from build123d import *

# Parameters (mm, degrees)
SKETCH1_W           = 16
SKETCH1_H           = 26
BOSS_EXTRUDE1_DEPTH = 3.5
SKETCH2_W           = 16
SKETCH2_H           = 26
BOSS_EXTRUDE2_DEPTH = 3.5
SKETCH3_R           = 5
CUT_EXTRUDE1_DEPTH  = 2.5


with BuildPart() as part:
    # Sketch1 → Boss-Extrude1 (new body)
    with BuildSketch(Plane.XY):
        with Locations((8, 13)):
            Rectangle(SKETCH1_W, SKETCH1_H)
        with BuildLine():
            Line((13.25, 23.790620927), (13.25, 2.209379073))
            ThreePointArc((13.25, 2.209379073), (8, 1), (2.75, 2.209379073))
            Line((2.75, 2.209379073), (2.75, 23.790620927))
            ThreePointArc((2.75, 23.790620927), (8, 25), (13.25, 23.790620927))
        make_face(mode=Mode.SUBTRACT)
    extrude(amount=BOSS_EXTRUDE1_DEPTH)

    # Sketch2 → Boss-Extrude2 (add)
    with BuildSketch(Plane.XY.offset(3.5)):
        with Locations((8, 13)):
            Rectangle(SKETCH2_W, SKETCH2_H)
    extrude(amount=BOSS_EXTRUDE2_DEPTH)

    # Sketch3 → Cut-Extrude1 (cut)
    with BuildSketch(Plane(origin=(0, 0, 3.5), x_dir=(-1, 0, 0), z_dir=(0, 0, -1))):
        with Locations((-8, 13)):
            Circle(SKETCH3_R)
    extrude(amount=-CUT_EXTRUDE1_DEPTH, mode=Mode.SUBTRACT)


solid = part.part
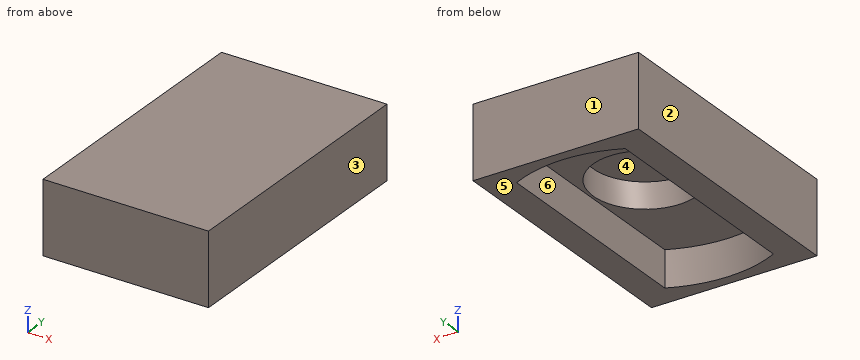
Verification items for the finished model (mm, model axes). Face numbers are marked on the shaded views. A direction names the side the tool comes from. Round coordinates to 2 decimals unless told otherwise and drop trailing zeros. Order: outer loops, then holes, each group sorted by start corner. A loop starts at its lowest first (then second) coordinate and runs counter-clockwise, first axis right, second up.
1. Access from +Z, -Z, +X, -X, +Y, -Y to the whole of each face (thin tool, end or side, straight path). Record for the marked faces 5 and 6.
Final values:
face 5: -Z, +X, -X, +Y, -Y
face 6: -Z
2. Section check D-D on y = 22.25. Record the cut outline in (x, z).
Final values:
outline: (0, 0) - (2.75, 0) - (2.75, 3.5) - (13.25, 3.5) - (13.25, 0) - (16, 0) - (16, 7) - (0, 7) - close
3. Go/stop test with flat-tipped pins: P1, Ø5, axis at x = 7, y = 12.5, coming from the -Z side; P2, Ø3, axis at x = 11.5, y = 10.5, coming from the -Z side. Record where each tip stops, or that it passes through.
Final values:
P1: stops at z = 6
P2: stops at z = 3.5
4. Section check B-B on z = 2.75. Record the cut outline in (x, y).
Final values:
outline: (0, 0) - (16, 0) - (16, 26) - (0, 26) - close; hole (2.75, 2.21) arc R12 ccw to (13.25, 2.21) - (13.25, 23.79) arc R12 ccw to (2.75, 23.79) - close
5. Section check A-A on y = 13. Record the cut outline in (x, z), then the cut area to 4 significant figures.
Final values:
outline: (0, 0) - (2.75, 0) - (2.75, 3.5) - (3, 3.5) - (3, 6) - (13, 6) - (13, 3.5) - (13.25, 3.5) - (13.25, 0) - (16, 0) - (16, 7) - (0, 7) - close
area: 50.25 mm2
6. Release check for a two-part mould opening along X. For the marked faces 1, 2, 3 and 4 record: +X half, -X half, draft (parallel to the pull), parting line (faces both ways), or undercut.
Final values:
face 1: draft
face 2: -X half
face 3: +X half
face 4: undercut
7. Section check C-C on x = 8. Record the cut outline in (y, z), then the cut area to 3 significant figures.
Final values:
outline: (0, 0) - (1, 0) - (1, 3.5) - (8, 3.5) - (8, 6) - (18, 6) - (18, 3.5) - (25, 3.5) - (25, 0) - (26, 0) - (26, 7) - (0, 7) - close
area: 73.0 mm2
8. Thickness scan on L1, parallel to Y at x = 8, z = 5.15; L2, parallel to X at y = 17, z = 2; L3, parallel to Z at x = 6.5, y = 20.5. Record the ranges inside material, lowest first.
Final values:
L1: y = 0 to 8, 18 to 26
L2: x = 0 to 2.75, 13.25 to 16
L3: z = 3.5 to 7
